Check sheet for the modelled part. Datum: model origin and axes. Units: mm. A direction names the side the tool comes from. Round coordinates to 2 decimals unless told otherwise and drop trailing zeros. Loops run counter-clockwise (first coordinate to the right, second up) from the corner with the lowest first, then second, coordinate; pieces in that order, holes last. Notation, with made-up numbers: M 6,-35.75 L 11,-35.75 A24 cw 11,-8.75 Z; hole C 20.25,-6.5 d9. An arc over 180 degrees is marked long. Write item = value, one per line. Start each with the question number.
(1) Cross-section at A-A on x = -7.5. Record the boundary of the cut face in (y, z), plus the area to 3 significant figures.
(2) Cross-section at C-C on z = 5. Record the boundary of the cut face in (x, y), plus the area to 3 significant figures.
(3) Go/stop test with flat-tipped pins: P1, Ø3, axis at y = 33.5, z = 3.5, coming from the -X side; P2, Ø12, axis at y = 8.5, z = 1.5, coming from the -X side; P3, Ø12, axis at x = -13, y = 31.5, coming from the -Z side; P4, Ø12, axis at y = -1, z = -5.5, coming from the +X side. Record where each tip stops, or that it passes through.
(4) Cross-section at D-D on y = 25. Record the boundary of the cut face in (x, z), plus the area to 3 significant figures.
(5) Cross-section at B-B on x = 60.5. Record the boundary of the cut face in (y, z), plus the area to 3 significant figures.
(6) Set-up check for faces 1 (the face through (-10, 5.5, 0)), 2 (the face through (56, 57.5, 0)), 3 (the face through (0, 7, 0)), 4 (the face through (-37.496, 24.615, 0.196)), 5 (the face through (-39.495, 24.571, -0.14)): record each of +Z, -Z, +X, -X, +Y, -Y from which the full face is reachable in a straight line by a thin tool's end or side.
(7) Mould release check, pull along Z, two halves, no side actions. Record for faces 6 (the face through (56, 44.5, 0)), 7 (the face through (18, 44, 14)), 8 (the face through (-10, 7.5, 0)): pulls with the +Z half, pulls with the -Z half, needs draft (parallel to the pull), parting line crosses it, or undercut.
(8) Scan lines: L1, parallel to Y at x = 6, z = -9.25; L2, parallel to Y at x = -35, z = -2; L3, parallel to X at y = 30.5, z = 4.75. Record each from-to range of solid material in increasing order. Write a range as from..to.
from build123d import *

# Parameters (mm, degrees)
SKETCH2_W   = 28
SKETCH2_H   = 15
SKETCH2_W_2 = 20
SKETCH2_H_2 = 11


with BuildPart() as part:
    # Sweep1: sweep along a path in Sketch1
    with BuildLine(Plane.XY) as sweep1_path:
        Line((0, 0), (-20, 0))
        ThreePointArc((-20, 0), (-45, 25), (-20, 50))
        Line((-20, 50), (130, 50))
    # Sketch2 → Sweep1 (sweep)
    with BuildSketch(Plane(origin=(0, 0, 0), x_dir=(0, 0, -1), z_dir=(1, 0, 0))):
        Rectangle(SKETCH2_W, SKETCH2_H)
        Rectangle(SKETCH2_W_2, SKETCH2_H_2, mode=Mode.SUBTRACT)
    sweep(path=sweep1_path.line)


solid = part.part
Result:
q1.outline = M -7.5,-14 L 7.5,-14 L 7.5,14 L -7.5,14 Z; M 42.5,-14 L 57.5,-14 L 57.5,14 L 42.5,14 Z; hole M -5.5,-10 L 5.5,-10 L 5.5,10 L -5.5,10 Z; hole M 44.5,-10 L 55.5,-10 L 55.5,10 L 44.5,10 Z
q1.area = 400 mm^2
q2.outline = M -20,-7.5 L 0,-7.5 L 0,-5.5 L -20,-5.5 A30.5 cw -20,55.5 L 130,55.5 L 130,57.5 L -20,57.5 A32.5 ccw Z; M -20,5.5 L 0,5.5 L 0,7.5 L -20,7.5 A17.5 cw -20,42.5 L 130,42.5 L 130,44.5 L -20,44.5 A19.5 ccw Z
q2.area = 994 mm^2
q3.P1 = -51.74
q3.P2 = -50.76
q3.P3 = through
q3.P4 = 0
q4.outline = M -52.5,-14 L -37.5,-14 L -37.5,14 L -52.5,14 Z; hole M -50.5,-10 L -39.5,-10 L -39.5,10 L -50.5,10 Z
q4.area = 200 mm^2
q5.outline = M 42.5,-14 L 57.5,-14 L 57.5,14 L 42.5,14 Z; hole M 44.5,-10 L 55.5,-10 L 55.5,10 L 44.5,10 Z
q5.area = 200 mm^2
q6.face_1 = +X
q6.face_2 = +Z, -Z, +X, -X, +Y
q6.face_3 = +Z, -Z, +X, -Y
q6.face_4 = +Z, -Z, +X
q6.face_5 = none
q7.face_6 = undercut
q7.face_7 = pulls with the +Z half
q7.face_8 = needs draft
q8.L1 = 42.5..44.5, 55.5..57.5
q8.L2 = -3.83..-1.56, 12.54..15.99, 34.01..37.46, 51.56..53.83
q8.L3 = -52.03..-50, -38.71..-36.61
